Design review of the part shown in the three views and the two pictorial views. Dimensions are in mm from the part's minimum x, y and z. A direction names the side the tool comes from. Coordinates: 2 decimals unless noted, no trailing zeros. Order: outer loops, then holes, each group sorted by start corner. A loop starts at its lowest first (then second) coordinate and runs counter-clockwise, first axis right, second up. Notation, with made-up numbers: (36, -25.75) -> (90, -25.75) arc R11 cw to (90, -14.75) -> close; hole circle Ø5 at (46, 13.5). An arc over 180 degrees is marked (long way). Answer as a JSON object with one key per item and string values. Group by question number.
1) Add section A-A, the plane x = 12.5. Write out the cut boundary in (y, z), then the cut area to 4 significant figures.
2) Add section D-D, the plane y = 6. Write out the cut boundary in (x, z).
3) For pin 1 (1.5 mm diameter, centred on y = 4, z = 6, fed in from +X); pin 2 (13 mm diameter, centred on x = 12.5, z = 12.5, fed in from -Y); pin 3 (2 mm diameter, centred on x = 12, y = 7.5, fed in from +Z), all flat-tipped, find the tip position at first contact; note any pin that passes through.
4) Wall thickness on L1, parallel to X at y = 7, z = 12.5; L2, parallel to X at y = 11.35, z = 12.5: over which ranges is each line inside the solid? List them lowest first.
5) Add section C-C, the plane y = 1.5. Write out the cut boundary in (x, z).
6) Machinability: for the marked faces 5, 6 and 7, which of the approach directions +Z, -Z, +X, -X, +Y, -Y give a long, thin tool a straight path to every point of the face, cutting with its end or side? Answer none if there is none.
7) Draft analysis for pull direction X (two halves, no side actions). For the marked faces 1, 2, 3 and 4, state which applies: +X half, -X half, draft (parallel to the pull), parting line (faces both ways), or undercut.
8) Add section B-B, the plane z = 12.5. Write out the cut boundary in (x, y), then the cut area to 4 significant figures.
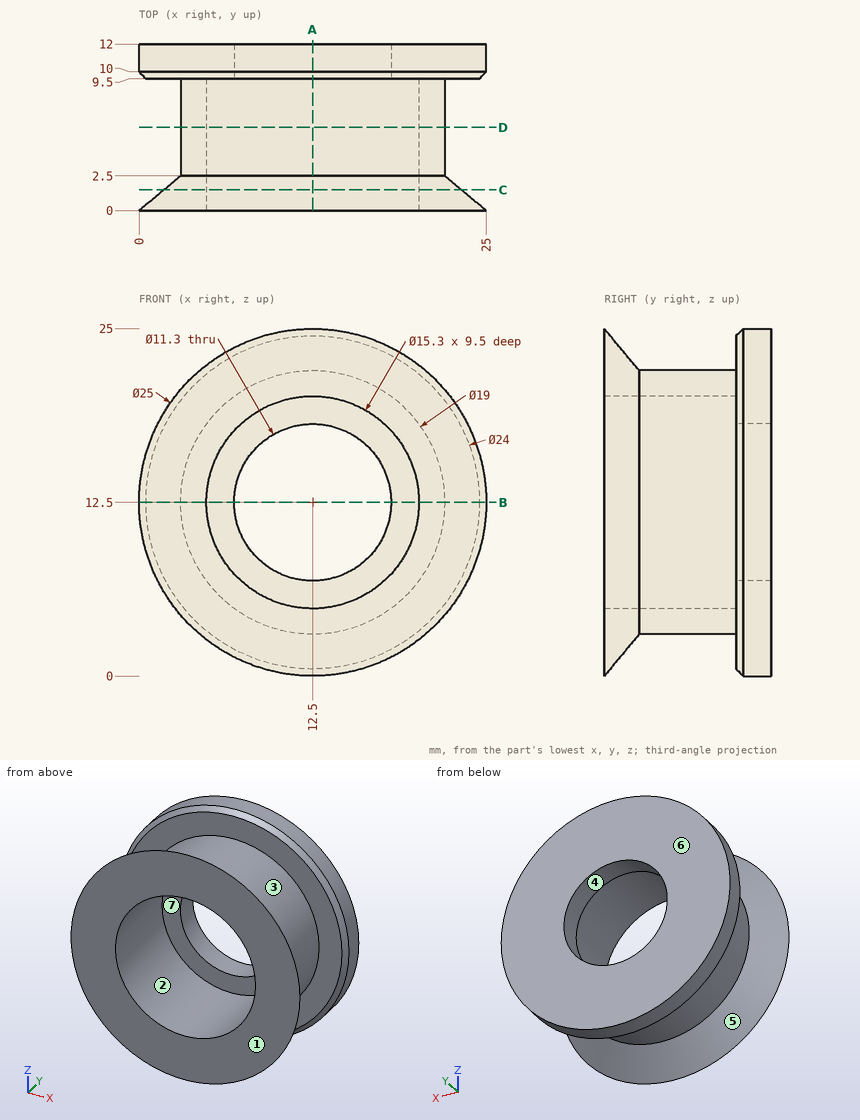
Output values:
{
 "1": {"outline": "(0, 0) -> (2.5, 3) -> (9.5, 3) -> (9.5, 0.5) -> (10, 0) -> (12, 0) -> (12, 6.85) -> (9.5, 6.85) -> (9.5, 4.85) -> (0, 4.85) -> close; (0, 20.15) -> (9.5, 20.15) -> (9.5, 18.15) -> (12, 18.15) -> (12, 25) -> (10, 25) -> (9.5, 24.5) -> (9.5, 22) -> (2.5, 22) -> (0, 25) -> close", "area": "76.65 mm²"},
 "2": {"outline": "circle Ø19 at (12.5, 12.5); hole circle Ø15.3 at (12.5, 12.5)"},
 "3": {"pin 1": "stops at x = 20.06", "pin 2": "stops at y = 9.5", "pin 3": "stops at z = 22"},
 "4": {"L1": "x = 3 to 4.85, 20.15 to 22", "L2": "x = 0 to 6.85, 18.15 to 25"},
 "5": {"outline": "circle Ø21.4 at (12.5, 12.5); hole circle Ø15.3 at (12.5, 12.5)"},
 "6": {"face 5": "none", "face 6": "+Z, -Z, +X, -X, +Y", "face 7": "-Y"},
 "7": {"face 1": "draft", "face 2": "undercut", "face 3": "parting line", "face 4": "undercut"},
 "8": {"outline": "(0, 0) -> (4.85, 0) -> (4.85, 9.5) -> (6.85, 9.5) -> (6.85, 12) -> (0, 12) -> (0, 10) -> (0.5, 9.5) -> (3, 9.5) -> (3, 2.5) -> close; (18.15, 9.5) -> (20.15, 9.5) -> (20.15, 0) -> (25, 0) -> (22, 2.5) -> (22, 9.5) -> (24.5, 9.5) -> (25, 10) -> (25, 12) -> (18.15, 12) -> close", "area": "76.65 mm²"}
}
